Geometry: final body of the model. Coordinates: model frame, mm. A direction names the side the tool comes from. Round coordinates to 2 decimals unless told otherwise and drop trailing zeros. Write each loop counter-clockwise with the first axis right and the second up, starting at its lowest first coordinate (ties: lowest second). Pieces come first, ordered by that corner, then holes. Notation, with made-up numbers: (50.5, 61) - (62.5, 61) arc R15 ccw to (62.5, 78) - close; hole circle Ø8 at (74, 40.5). An arc over 180 degrees is marked (long way). Write each question's results on one line, items separated by ' | '.
from build123d import *

# Parameters (mm, degrees)
EXTRUDE_1_DEPTH     = 110
SKETCH_3_R          = 1.35
CUT_EXTRUDE_2_DEPTH = 110
CUT_EXTRUDE_3_DEPTH = 65
SKETCH1_R           = 0.785
SKETCH1_R_2         = 1
SKETCH1_R_3         = 1.05
CUT_EXTRUDE1_DEPTH  = 10
SKETCH2_W           = 70.969328166
SKETCH2_H           = 159.698844539
CUT_EXTRUDE2_DEPTH  = 10
BOSS_EXTRUDE1_DEPTH = 5.5
SKETCH4_R           = 1.6
CUT_EXTRUDE3_DEPTH  = 20
CHAMFER1_SIZE       = 6.5
SKETCH5_R           = 7.5
CUT_EXTRUDE4_DEPTH  = 10


with BuildPart() as part:
    # 草图1 → 凸台-拉伸1 (new body)
    with BuildSketch(Plane(origin=(0, 0, 0), x_dir=(1, 0, 0), z_dir=(0, 1, 0))):
        Polygon((-46.858999723, -0.34362784), (-46.858999723, 2.65637216), (-24.358999723, -0.08362784), (-6.358999723, -0.08362784), (16.141000277, 2.660274599), (16.141000277, -0.34362784), (16.141000277, -3.08362784), (-6.358999723, -3.08362784), (-24.358999723, -3.08362784), (-46.858999723, -3.08362784), align=None)
    extrude(amount=EXTRUDE_1_DEPTH)

    # 草图3 → 切除-拉伸2 (cut)
    with BuildSketch(Plane.XY.offset(3.08362784)):
        with Locations((11.641000277, 90)):
            Circle(SKETCH_3_R)
        with Locations((11.641000277, 20.7)):
            Circle(SKETCH_3_R)
        with Locations((-42.358999723, 20.7)):
            Circle(SKETCH_3_R)
        with Locations((-42.358999723, 90)):
            Circle(SKETCH_3_R)
    extrude(amount=-CUT_EXTRUDE_2_DEPTH, mode=Mode.SUBTRACT)

    # 草图4 → 切除-拉伸3 (cut)
    with BuildSketch(Plane(origin=(0, 0, 0.08362784), x_dir=(-1, 0, 0), z_dir=(0, 0, -1))):
        Polygon((40.908999723, 6.9), (40.908999723, 13.2), (47.093892861, 16.7), (47.093892861, 24.7), (40.908999723, 28.2), (40.908999723, 82.5), (47.093892861, 86), (47.093892861, 94), (40.908999723, 97.5), (40.908999723, 103.8), (-10.191000277, 103.8), (-10.191000277, 97.5), (-16.375893416, 94), (-16.375893416, 86), (-10.191000277, 82.5), (-10.191000277, 28.2), (-16.375893416, 24.7), (-16.375893416, 16.7), (-10.191000277, 13.2), (-10.191000277, 6.9), align=None)
    extrude(amount=CUT_EXTRUDE_3_DEPTH, mode=Mode.SUBTRACT)

    # Sketch1 → Cut-Extrude1 (cut)
    with BuildSketch(Plane.XY.offset(3.08362784)):
        with Locations((-42.558897723, 106.265557005)):
            Circle(SKETCH1_R)
        with Locations((-39.858893724, 103.999988001)):
            Circle(SKETCH1_R_2)
        with Locations((-22.358833723, 105)):
            Circle(SKETCH1_R_2)
        with Locations((-22.358833723, 25)):
            Circle(SKETCH1_R_2)
        with Locations((-39.858893724, 27.999986001)):
            Circle(SKETCH1_R_3)
        with Locations((-41.358999723, 23.749988001)):
            Circle(SKETCH1_R)
        with Locations((-41.358999723, 7.749988001)):
            Circle(SKETCH1_R)
        with Locations((-25.358999723, 7.749988001)):
            Circle(SKETCH1_R)
        with Locations((-5.358999723, 7.749988001)):
            Circle(SKETCH1_R)
        with Locations((10.641000277, 7.749988001)):
            Circle(SKETCH1_R)
        with Locations((10.641000277, 23.749988001)):
            Circle(SKETCH1_R)
        with Locations((9.140894279, 27.999986001)):
            Circle(SKETCH1_R_3)
        with Locations((-8.359165723, 25)):
            Circle(SKETCH1_R_2)
        with Locations((-8.359165723, 105)):
            Circle(SKETCH1_R_2)
        with Locations((9.140894279, 103.999988001)):
            Circle(SKETCH1_R_2)
        with Locations((11.840898278, 106.265557005)):
            Circle(SKETCH1_R)
    extrude(amount=-CUT_EXTRUDE1_DEPTH, mode=Mode.SUBTRACT)

    # Sketch2 → Cut-Extrude2 (cut)
    with BuildSketch(Plane(origin=(0, 0, -2.41637216), x_dir=(-1, 0, 0), z_dir=(0, 0, -1))):
        with Locations((16.341269992, 58.054935109)):
            Rectangle(SKETCH2_W, SKETCH2_H)
    extrude(amount=CUT_EXTRUDE2_DEPTH, mode=Mode.SUBTRACT)

    # Sketch3 → Boss-Extrude1 (add)
    with BuildSketch(Plane.XY.offset(3.08362784)):
        Polygon((-46.858999723, 85), (-56.858999723, 75), (-56.858999723, 35), (-46.858999723, 25), align=None)
        Polygon((16.141000277, 85), (16.141000277, 25), (26.141000277, 35), (26.141000277, 75), align=None)
    extrude(amount=-BOSS_EXTRUDE1_DEPTH)

    # Sketch4 → Cut-Extrude3 (cut)
    with BuildSketch(Plane(origin=(0, 0, -2.41637216), x_dir=(-1, 0, 0), z_dir=(0, 0, -1))):
        with Locations((-21.141000277, 74)):
            Circle(SKETCH4_R)
        with Locations((-21.141000277, 36)):
            Circle(SKETCH4_R)
        with Locations((51.858999723, 74)):
            Circle(SKETCH4_R)
        with Locations((51.858999723, 36)):
            Circle(SKETCH4_R)
    extrude(amount=-CUT_EXTRUDE3_DEPTH, mode=Mode.SUBTRACT)

    # Chamfer1
    chamfer1_edges = [part.edges().sort_by_distance(p)[0] for p in [
        (16.141000277, 110, 0.33362784),
        (-46.858999723, 110, 0.33362784),
        (16.141000277, 0, 0.33362784),
        (-46.858999723, 0, 0.33362784),
    ]]
    chamfer(chamfer1_edges, length=CHAMFER1_SIZE)

    # Sketch5 → Cut-Extrude4 (cut)
    with BuildSketch(Plane(origin=(0, 0, 0.08362784), x_dir=(-1, 0, 0), z_dir=(0, 0, -1))):
        with Locations((31.858999723, 17)):
            Circle(SKETCH5_R)
        with Locations((-1.141000277, 17)):
            Circle(SKETCH5_R)
        with BuildLine():
            Line((28.858999723, 32), (1.858999723, 32))
            ThreePointArc((1.858999723, 32), (-1.141000277, 35), (1.858999723, 38))
            Line((1.858999723, 38), (28.858999723, 38))
            ThreePointArc((28.858999723, 38), (31.858999723, 35), (28.858999723, 32))
        make_face()
        with BuildLine():
            Line((28.858999723, 42), (1.858999723, 42))
            ThreePointArc((1.858999723, 42), (-1.141000277, 45), (1.858999723, 48))
            Line((1.858999723, 48), (28.858999723, 48))
            ThreePointArc((28.858999723, 48), (31.858999723, 45), (28.858999723, 42))
        make_face()
        with BuildLine():
            Line((28.858999723, 52), (1.858999723, 52))
            ThreePointArc((1.858999723, 52), (-1.141000277, 55), (1.858999723, 58))
            Line((1.858999723, 58), (28.858999723, 58))
            ThreePointArc((28.858999723, 58), (31.858999723, 55), (28.858999723, 52))
        make_face()
        with BuildLine():
            Line((28.858999723, 62), (1.858999723, 62))
            ThreePointArc((1.858999723, 62), (-1.141000277, 65), (1.858999723, 68))
            Line((1.858999723, 68), (28.858999723, 68))
            ThreePointArc((28.858999723, 68), (31.858999723, 65), (28.858999723, 62))
        make_face()
        with BuildLine():
            Line((28.858999723, 72), (1.858999723, 72))
            ThreePointArc((1.858999723, 72), (-1.141000277, 75), (1.858999723, 78))
            Line((1.858999723, 78), (28.858999723, 78))
            ThreePointArc((28.858999723, 78), (31.858999723, 75), (28.858999723, 72))
        make_face()
        with BuildLine():
            Line((28.858999723, 82), (1.858999723, 82))
            ThreePointArc((1.858999723, 82), (-1.141000277, 85), (1.858999723, 88))
            Line((1.858999723, 88), (28.858999723, 88))
            ThreePointArc((28.858999723, 88), (31.858999723, 85), (28.858999723, 82))
        make_face()
        with BuildLine():
            Line((28.858999723, 92), (1.858999723, 92))
            ThreePointArc((1.858999723, 92), (-1.141000277, 95), (1.858999723, 98))
            Line((1.858999723, 98), (28.858999723, 98))
            ThreePointArc((28.858999723, 98), (31.858999723, 95), (28.858999723, 92))
        make_face()
    extrude(amount=-CUT_EXTRUDE4_DEPTH, mode=Mode.SUBTRACT)


solid = part.part
Q1. Pin query (flat end, axial travel): pin 1 (2 mm diameter, centred on y = 11.5, z = -0.5, fed in from +X); pin 2 (2.5 mm diameter, centred on x = -41.36, y = 7.75, fed in from -Z); pin 3 (0.9 mm diameter, centred on x = -42.56, y = 106.27, fed in from -Z); pin 4 (2.5 mm diameter, centred on x = -41.36, y = 23.75, fed in from -Z). Return the tip coordinate at first contact, or that it passes through.
Answer block:
pin 1: x = 16.14 | pin 2: z = -2.14 | pin 3: through | pin 4: z = 0.08
Q2. Section query D-D, the plane z = 1.9. Give the number of separate pieces and of enclosed holes in the cut face, plus the area to 3 significant figures.
Answer block:
separate pieces: 1 | enclosed holes: 33 | area: 6,060 mm2
Q3. Access query for faces 4 (the flat face through (-42.926, 54.938, -2.177)), 5 (the flat face through (16.141, 96, 1)), 6 (the flat face through (-43.84, 84.16, -1.15)). Directions: +Z, -Z, +X, -X, +Y, -Y. A direction counts if a zero-diameter tool reaches every point of the face in a straight line with its end or side. Return the directions, or none.
Answer block:
face 4: -Z, +Y, -Y | face 5: +Z, -Z, +X, +Y | face 6: -Z
Q4. Section query A-A, the plane y = 55. Return loops of the section in (x, z), plus the area to 3 significant figures.
Answer block:
outline: (-56.86, -2.42) - (-44.89, -2.42) - (-40.91, -1.93) - (-40.91, 0.08) - (-31.86, 0.08) - (-31.86, 3.08) - (-56.86, 3.08) - close; (1.14, 0.08) - (10.19, 0.08) - (10.19, -1.93) - (14.14, -2.42) - (26.14, -2.42) - (26.14, 3.08) - (1.14, 3.08) - close | area: 228 mm2
Q5. Section query B-B, the plane y = 90. Return loops of the section in (x, z), plus the area to 3 significant figures.
Answer block:
outline: (-46.86, 0.08) - (-43.71, 0.08) - (-43.71, 3.08) - (-46.86, 3.08) - close; (-41.01, 0.08) - (10.29, 0.08) - (10.29, 3.08) - (-41.01, 3.08) - close; (12.99, 0.08) - (16.14, 0.08) - (16.14, 3.08) - (12.99, 3.08) - close | area: 173 mm2
Q6. Section query C-C, the plane y = 101.5. Return loops of the section in (x, z), plus the area to 3 significant figures.
Answer block:
outline: (-46.86, -2.42) - (-44.89, -2.42) - (-40.91, -1.93) - (-40.91, 0.08) - (10.19, 0.08) - (10.19, -1.93) - (14.14, -2.42) - (16.14, -2.42) - (16.14, 3.08) - (-46.86, 3.08) - close | area: 217 mm2
Q7. Ray query, line 1 along Y through (x, z) = (1.5, -0.35); line 2 along Y through (x, z) = (22, -1.35); line 3 along X through (y, z) = (101, -0.85). Return the intervals inside material, ascending.
Answer block:
line 1: 0 to 6.9, 103.8 to 110 | line 2: 30.86 to 34.65, 37.35 to 72.65, 75.35 to 79.14 | line 3: -46.86 to -40.91, 10.19 to 16.14
Q8. Mould query, pull axis X, two halves, no side actions, for faces 1 (the cylindrical face through (-31.86, 95.07, 1.56)), 2 (the flat face through (-34, 54, 3.084)), 3 (the flat face through (12.94, 3.3, 0.37)). Classes: pulls with the +X half, pulls with the -X half, needs draft (parallel to the pull), parting line crosses it, or undercut.
Answer block:
face 1: undercut | face 2: needs draft | face 3: pulls with the +X half
